```python
from build123d import *

# Parameters (mm, degrees)
F1_DEPTH = 30
F2_W     = 30
F2_H     = 30
F3_DEPTH = 20


with BuildPart() as f1:
    # F0 (on Front) → F1 (new body)
    with BuildSketch(Plane.XZ):
        Polygon((0, 10), (0, 0), (30, 0), (30, -30), (70, -30), (70, 10), align=None)
    extrude(amount=F1_DEPTH)

    # F2 (on face) → F3 (cut)
    with BuildSketch(Plane.XZ.offset(30)):
        with Locations((55, -5)):
            Rectangle(F2_W, F2_H)
    extrude(amount=-F3_DEPTH, mode=Mode.SUBTRACT)


solid = f1.part
```
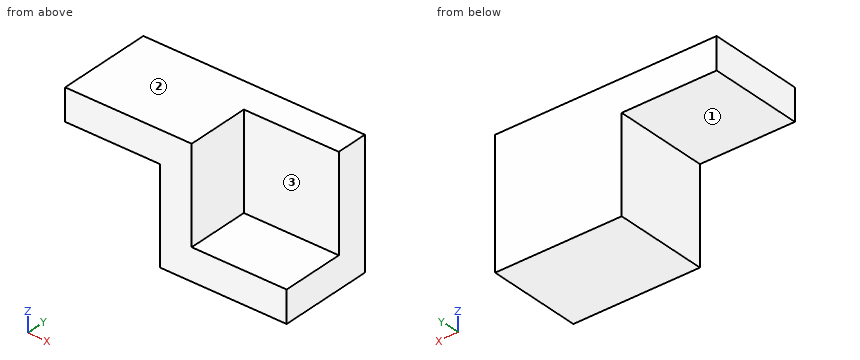
CAD build for the part. Positions are in the model's coordinates, mm. Face numbers are marked on the shaded views. A direction names the side the tool comes from. Give positions to 0.01 mm unless a question says otherwise; leave off trailing zeros. Order: outer loops, then holes, each group sorted by start corner. A loop starts at its lowest first (then second) coordinate and runs counter-clockwise, first axis right, second up.
(1) Saw through at D-D, the plane x = 14. Give the cut face in (y, z), then the cut area to 3 significant figures.
(2) Drill centre lines: L1, parallel to Z at x = 64, y = -11.75; L2, parallel to X at y = -13, z = -12; L3, parallel to Y at x = 59, z = -11.5. Where is each one in solid material? Low to high.
(3) Saw through at A-A, the plane z = -8.5. Give the cut face in (x, y), then the cut area to 3 significant figures.
(4) Saw through at C-C, the plane x = 52.5. Give the cut face in (y, z), then the cut area to 3 significant figures.
(5) Tool access for the marked faces 1, 2 and 3: list every direction of +Z, -Z, +X, -X, +Y, -Y with a clear straight run to the whole face (end or side of a thin tool).
(6) Saw through at B-B, the plane y = -25.75. Give the cut face in (x, z).
(7) Flat gauge pins, fed straight in: pin 1 (2 mm diameter, centred on x = 7.5, y = -3, fed in from -Z); pin 2 (16 mm diameter, centred on y = -22.5, z = -7, fed in from +X); pin 3 (2 mm diameter, centred on x = 51.5, y = -19.5, fed in from +Z). Where does each tip first touch, or does it go through?
Results found:
1. outline: (-30, 0) - (0, 0) - (0, 10) - (-30, 10) - close
1. area: 300 mm2
2. L1: z = -30 to -20
2. L2: x = 30 to 40
2. L3: y = -10 to 0
3. outline: (30, -30) - (40, -30) - (40, -10) - (70, -10) - (70, 0) - (30, 0) - close
3. area: 600 mm2
4. outline: (-30, -30) - (0, -30) - (0, 10) - (-10, 10) - (-10, -20) - (-30, -20) - close
4. area: 600 mm2
5. face 1: -Z, -X, +Y, -Y
5. face 2: +Z, +X, -X, +Y, -Y
5. face 3: +Z, +X, -Y
6. outline: (0, 0) - (30, 0) - (30, -30) - (70, -30) - (70, -20) - (40, -20) - (40, 10) - (0, 10) - close
7. pin 1: stops at z = 0
7. pin 2: stops at x = 40
7. pin 3: stops at z = -20
